Could you check a few things on this model? Use its own coordinates, in mm. A direction names the side the tool comes from. Coordinates: 2 decimals unless noted, no trailing zeros. Write each loop counter-clockwise with the first axis right and the second up, starting at its lowest first coordinate (ties: lowest second). Pieces come first, ordered by that corner, then holes.
```python
from build123d import *

# Parameters (mm, degrees)
F1_DEPTH     = 76.2
F2_W         = 83.8339800673
F2_H         = 0.635
F3_DEPTH     = 76.201
F4_W         = 71.12
F4_H         = 79.6544
F5_DEPTH     = 1.27
F6_R         = 5.08
F7_T1_DEPTH  = 33.7228350816
F7_S5_W      = 5.08
F7_S5_H      = 5.08
F7_T6_DEPTH  = 5.08
F8_T1_DEPTH  = 33.7228350816
F8_S5_W      = 5.08
F8_S5_H      = 5.08
F8_T6_DEPTH  = 5.08
F9_T1_DEPTH  = 33.7228350816
F9_S5_W      = 5.08
F9_S5_H      = 5.08
F9_T6_DEPTH  = 5.08
F10_T1_DEPTH = 33.7228350816
F10_S5_W     = 5.08
F10_S5_H     = 5.08
F10_T6_DEPTH = 5.08


# Not quite as in the source:
# - a fillet or chamfer that OpenCascade refuses, or shapes differently, is made with other operations: its cross-section is extruded or revolved along the edge and cut away or added


with BuildPart() as f1:
    # F0 (on Right) → F1 (new body)
    with BuildSketch(Plane.YZ):
        Polygon((0, 26.1028350816), (0, 0), (2.54, 0), (2.54, 12.7), (86.36, 12.7), (86.36, 0), (88.9, 0), (88.9, 26.1028350816), align=None)
    extrude(amount=-F1_DEPTH)

    # F2 (on face) → F3 (cut, through all)
    with BuildSketch(Plane.YZ):
        with Locations((44.4430099664, 13.6525)):
            Rectangle(F2_W, F2_H)
    extrude(amount=-F3_DEPTH, mode=Mode.SUBTRACT)

    # F4 (on face) → F5 (cut)
    with BuildSketch(Plane(origin=(0, 0, 12.7), x_dir=(1, 0, 0), z_dir=(0, 0, -1))):
        with Locations((-38.1, -44.45)):
            Rectangle(F4_W, F4_H)
    extrude(amount=-F5_DEPTH, mode=Mode.SUBTRACT)

    # F6
    f6_edges = [f1.edges().sort_by_distance(p)[0] for p in [
        (-38.1, 0, 26.102835),
        (0, 44.45, 26.102835),
        (-38.1, 88.9, 26.102835),
        (-76.2, 44.45, 26.102835),
    ]]
    fillet(f6_edges, radius=F6_R)

    # F7: fillet of radius 5.08 on 1 edges, made by hand

    # F7_s2 → F7_t1 (cut)
    with BuildSketch(Plane.XY.offset(-12.7)):
        with BuildLine():
            ThreePointArc((-5.08, 0), (-1.4878975516, 1.4878975516), (0, 5.08))
            Line((0, 5.08), (0, 0))
            Line((0, 0), (-5.08, 0))
        make_face()
    extrude(amount=F7_T1_DEPTH, mode=Mode.SUBTRACT)


with BuildPart() as f7_tool4:
    # F7_s5 → F7_t6 (new body)
    with BuildSketch(Plane.XZ.offset(-5.08)):
        with Locations((-2.54, 23.5628350816)):
            Rectangle(F7_S5_W, F7_S5_H)
    extrude(amount=F7_T6_DEPTH)

    # F7_s7 → F7_t8 (revolve, cut)
    with BuildSketch(Plane(origin=(-5.08, 5.08, 21.0228350816), x_dir=(-0.7071067812, 0, -0.7071067812), z_dir=(-0.7071067812, 0, 0.7071067812))):
        with BuildLine():
            ThreePointArc((0, -5.08), (5.08, 0), (0, 5.08))
            Line((0, 5.08), (0, -5.08))
        make_face()
    revolve(axis=Axis((-5.08, 5.08, 21.0228350816), (0, -1, 0)), mode=Mode.SUBTRACT)


with BuildPart() as f1_1:
    add(f1.part)

    # F7_t3: cut F7_tool4
    add(f7_tool4.part, mode=Mode.SUBTRACT)

    # F8: fillet of radius 5.08 on 1 edges, made by hand

    # F8_s2 → F8_t1 (cut)
    with BuildSketch(Plane.XY.offset(-12.7)):
        with BuildLine():
            ThreePointArc((0, 83.82), (-1.4878975516, 87.4121024484), (-5.08, 88.9))
            Line((-5.08, 88.9), (0, 88.9))
            Line((0, 88.9), (0, 83.82))
        make_face()
    extrude(amount=F8_T1_DEPTH, mode=Mode.SUBTRACT)


with BuildPart() as f8_tool4:
    # F8_s5 → F8_t6 (new body)
    with BuildSketch(Plane.YZ.offset(-5.08)):
        with Locations((86.36, 23.5628350816)):
            Rectangle(F8_S5_W, F8_S5_H)
    extrude(amount=F8_T6_DEPTH)

    # F8_s7 → F8_t8 (revolve, cut)
    with BuildSketch(Plane(origin=(-5.08, 83.82, 21.0228350816), x_dir=(0, -0.7071067812, -0.7071067812), z_dir=(0, -0.7071067812, 0.7071067812))):
        with BuildLine():
            ThreePointArc((0, -5.08), (5.08, 0), (0, 5.08))
            Line((0, 5.08), (0, -5.08))
        make_face()
    revolve(axis=Axis((-5.08, 83.82, 21.0228350816), (1, 0, 0)), mode=Mode.SUBTRACT)


with BuildPart() as f1_2:
    add(f1_1.part)

    # F8_t3: cut F8_tool4
    add(f8_tool4.part, mode=Mode.SUBTRACT)

    # F9: fillet of radius 5.08 on 1 edges, made by hand

    # F9_s2 → F9_t1 (cut)
    with BuildSketch(Plane.XY.offset(-12.7)):
        with BuildLine():
            ThreePointArc((-71.12, 0), (-74.7121024484, 1.4878975516), (-76.2, 5.08))
            Line((-76.2, 5.08), (-76.2, 0))
            Line((-76.2, 0), (-71.12, 0))
        make_face()
    extrude(amount=F9_T1_DEPTH, mode=Mode.SUBTRACT)


with BuildPart() as f9_tool4:
    # F9_s5 → F9_t6 (new body)
    with BuildSketch(Plane.XZ.offset(-5.08)):
        with Locations((-73.66, 23.5628350816)):
            Rectangle(F9_S5_W, F9_S5_H)
    extrude(amount=F9_T6_DEPTH)

    # F9_s7 → F9_t8 (revolve, cut)
    with BuildSketch(Plane(origin=(-71.12, 5.08, 21.0228350816), x_dir=(0.7071067812, 0, -0.7071067812), z_dir=(-0.7071067812, 0, -0.7071067812))):
        with BuildLine():
            ThreePointArc((0, -5.08), (5.08, 0), (0, 5.08))
            Line((0, 5.08), (0, -5.08))
        make_face()
    revolve(axis=Axis((-71.12, 5.08, 21.0228350816), (0, -1, 0)), mode=Mode.SUBTRACT)


with BuildPart() as f1_3:
    add(f1_2.part)

    # F9_t3: cut F9_tool4
    add(f9_tool4.part, mode=Mode.SUBTRACT)

    # F10: fillet of radius 5.08 on 1 edges, made by hand

    # F10_s2 → F10_t1 (cut)
    with BuildSketch(Plane.XY.offset(-12.7)):
        with BuildLine():
            ThreePointArc((-76.2, 83.82), (-74.7121024484, 87.4121024484), (-71.12, 88.9))
            Line((-71.12, 88.9), (-76.2, 88.9))
            Line((-76.2, 88.9), (-76.2, 83.82))
        make_face()
    extrude(amount=F10_T1_DEPTH, mode=Mode.SUBTRACT)


with BuildPart() as f10_tool4:
    # F10_s5 → F10_t6 (new body)
    with BuildSketch(Plane.YZ.offset(-71.12)):
        with Locations((86.36, 23.5628350816)):
            Rectangle(F10_S5_W, F10_S5_H)
    extrude(amount=-F10_T6_DEPTH)

    # F10_s7 → F10_t8 (revolve, cut)
    with BuildSketch(Plane(origin=(-71.12, 83.82, 21.0228350816), x_dir=(0, -0.7071067812, -0.7071067812), z_dir=(0, 0.7071067812, -0.7071067812))):
        with BuildLine():
            ThreePointArc((0, -5.08), (5.08, 0), (0, 5.08))
            Line((0, 5.08), (0, -5.08))
        make_face()
    revolve(axis=Axis((-71.12, 83.82, 21.0228350816), (-1, 0, 0)), mode=Mode.SUBTRACT)


with BuildPart() as f1_4:
    add(f1_3.part)

    # F10_t3: cut F10_tool4
    add(f10_tool4.part, mode=Mode.SUBTRACT)


solid = f1_4.part
```
1. I want a section at B-B on y = 58.5. Please give me the cut outline in (x, z) (3 decimals).
Verdict:
outline: (-76.2, 12.7) - (-73.66, 12.7) - (-73.66, 13.335) - (-76.2, 13.335) - close; (-76.2, 13.97) - (0, 13.97) - (0, 21.023) arc R5.08 ccw to (-5.08, 26.103) - (-71.12, 26.103) arc R5.08 ccw to (-76.2, 21.023) - close; (-2.54, 12.7) - (0, 12.7) - (0, 13.335) - (-2.54, 13.335) - close
2. If we mould it in two halves opening along Z, with no side actions, what happens to faces 3 (the face through (-1.528, 43.899, 24.654)), 4 (the face through (-38, 1, 0)), 5 (the face through (-38, 86.36, 6)), 6 (the face through (-75, 41, 13.335))? For each: pulls with the +Z half, pulls with the -Z half, needs draft (parallel to the pull), parting line crosses it, or undercut.
Verdict:
face 3: pulls with the +Z half
face 4: pulls with the -Z half
face 5: needs draft
face 6: undercut
3. Please list where these lines run through material, in increasing order: line 1 along Y through (x, z) = (-37, 10.25); line 2 along Y through (x, z) = (-61, 12.75); line 3 along Z through (x, y) = (-60, 59).
Verdict:
line 1: y = 0 to 2.54, 86.36 to 88.9
line 2: y = 0 to 4.62, 84.28 to 88.9
line 3: z = 13.97 to 26.1
4. I want a section at C-C on x = -56. Please give me the cut outline in (y, z) (3 decimals).
Verdict:
outline: (0, 0) - (2.54, 0) - (2.54, 12.7) - (4.623, 12.7) - (4.623, 13.335) - (2.526, 13.335) - (2.526, 13.97) - (86.36, 13.97) - (86.36, 13.335) - (84.277, 13.335) - (84.277, 12.7) - (86.36, 12.7) - (86.36, 0) - (88.9, 0) - (88.9, 21.023) arc R5.08 ccw to (83.82, 26.103) - (5.08, 26.103) arc R5.08 ccw to (0, 21.023) - close
5. I want a section at A-A on z = 10. Please give me the cut outline in (x, y).
Verdict:
outline: (-75.52, 2.54) arc R5.08 ccw to (-71.12, 0) - (-5.08, 0) arc R5.08 ccw to (-0.68, 2.54) - close; (-75.52, 86.36) - (-0.68, 86.36) arc R5.08 ccw to (-5.08, 88.9) - (-71.12, 88.9) arc R5.08 ccw to start
6. On a 3-axis mill with a long thin cutter (end or side, diameter ignored), from which of +Z, -Z, +X, -X, +Y, -Y can I reach the whole of each face in a straight line? I mean faces 1 (the face through (-75, 41, 12.7)), 2 (the face through (-38.562, 1.449, 24.575)). Say none if no direction works.
Verdict:
face 1: -Z, +X, -X
face 2: +Z, +X, -X, -Y
